```python
from build123d import *

# Parameters (mm, degrees)
F1_DEPTH  = 25
F2_R      = 4
F3_R      = 3.9581459444
F4_R      = 5
F6_DEPTH  = 4
F7_R      = 1
F9_DEPTH  = 10
F11_D     = 8.5
F11_DEPTH = 20
F11_TIP   = 2.5536576309
F13_D     = 10.3
F13_DEPTH = 4
F13_TIP   = 3.094432188
F15_D     = 10
F15_DEPTH = 4
F15_TIP   = 3.0043030951


with BuildPart() as f1:
    # F0 (on Front) → F1 (new body)
    with BuildSketch(Plane.XZ):
        Polygon((-11.592581531, 8.7356367638), (0, 0), (61, 0), (47.3139187714, 38.6483011348), (67.3029387003, 42.7151132025), (66.5054669627, 46.634812021), (42.0073493471, 41.6506136606), (55.3401309115, 4), (1.338381278, 4), (-10.3797117652, 12.8302164722), (-61.3117864463, 9.2686988641), (-61.0327605513, 5.278442663), align=None)
    extrude(amount=F1_DEPTH)

    # F2
    f2_edges = [f1.edges().sort_by_distance(p)[0] for p in [
        (42.007349, -12.5, 41.650614),
        (1.338381, -12.5, 4),
        (-10.379712, -12.5, 12.830216),
        (-11.592582, -12.5, 8.735637),
        (0, -12.5, 0),
        (47.313919, -12.5, 38.648301),
    ]]
    fillet(f2_edges, radius=F2_R)

    # F3
    f3_edges = [f1.edges().sort_by_distance(p)[0] for p in [
        (55.340131, -12.5, 4),
        (61, -12.5, 0),
    ]]
    fillet(f3_edges, radius=F3_R)

    # F4
    f4_edges = [f1.edges().sort_by_distance(p)[0] for p in [
        (66.904203, -25, 44.674963),
        (66.904203, 0, 44.674963),
    ]]
    fillet(f4_edges, radius=F4_R)

    # F5 (on face) → F6 (cut)
    with BuildSketch(Plane(origin=(-0.9433178269, 0, 13.4900734165), x_dir=(0.9975640503, 0, 0.0697564737), z_dir=(-0.0697564737, 0, 0.9975640503))):
        Polygon((-60.5158822671, 0), (-60.5158822671, -7.5), (-50.5158822671, -7.5), (-40.5158822671, 0), align=None)
        Polygon((-50.5158822671, -17.5), (-60.5158822671, -17.5), (-60.5158822671, -25), (-40.5158822671, -25), align=None)
    extrude(amount=-F6_DEPTH, mode=Mode.SUBTRACT)

    # F7
    f7_edges = [f1.edges().sort_by_distance(p)[0] for p in [
        (-41.220992, -25, 8.6687),
        (-51.196633, -17.5, 7.971136),
        (-61.172273, -17.5, 7.273571),
        (-61.172273, -7.5, 7.273571),
        (-41.220992, 0, 8.6687),
        (-51.196633, -7.5, 7.971136),
    ]]
    fillet(f7_edges, radius=F7_R)

    # F8 (on face) → F9 (join)
    with BuildSketch(Plane(origin=(-0.9433178269, 0, 13.4900734165), x_dir=(0.9975640503, 0, 0.0697564737), z_dir=(-0.0697564737, 0, 0.9975640503))):
        Polygon((-36.7410970494, -19.5), (-32.6996451651, -12.5), (-36.7410970494, -5.5), (-44.8240008181, -5.5), (-48.8654527024, -12.5), (-44.8240008181, -19.5), align=None)
    extrude(amount=F9_DEPTH)

    # F11
    with Locations(Plane(origin=(-1.6408825643, 0, 23.4657139191), x_dir=(0.9975640503, 0, 0.0697564737), z_dir=(-0.0697564737, 0, 0.9975640503))):
        with Locations((-40.7825489337, -12.5)):
            Hole(F11_D / 2, depth=F11_DEPTH)
            with Locations((0, 0, -(F11_DEPTH + F11_TIP / 2))):  # 118° drill point
                Cone(0, F11_D / 2, F11_TIP, mode=Mode.SUBTRACT)

    # F13
    with Locations(Plane(origin=(-0.6642919319, 0, 9.4998172155), x_dir=(0.9975640503, 0, 0.0697564737), z_dir=(0.0697564737, 0, -0.9975640503))):
        with Locations((-40.7825489337, 12.5)):
            Hole(F13_D / 2, depth=F13_DEPTH)
            with Locations((0, 0, -(F13_DEPTH + F13_TIP / 2))):  # 118° drill point
                Cone(0, F13_D / 2, F13_TIP, mode=Mode.SUBTRACT)

    # F15
    with Locations(Plane(origin=(-6.4674054427, 0, 31.7883133346), x_dir=(0.9799247046, 0, 0.1993679344), z_dir=(-0.1993679344, 0, 0.9799247046))):
        with Locations((64.4678362136, -14)):
            Hole(F15_D / 2, depth=F15_DEPTH)
            with Locations((0, 0, -(F15_DEPTH + F15_TIP / 2))):  # 118° drill point
                Cone(0, F15_D / 2, F15_TIP, mode=Mode.SUBTRACT)


solid = f1.part
```
CAD build for the part. Positions are in the model's coordinates, mm. A direction names the side the tool comes from. Coordinates: 2 decimals unless noted, no trailing zeros. Order: outer loops, then holes, each group sorted by start corner. A loop starts at its lowest first (then second) coordinate and runs counter-clockwise, first axis right, second up. Notation, with made-up numbers: (-17, -24) -> (25, -24) arc R22 cw to (25, 1) -> close; hole circle Ø7 at (-13, -38). An arc over 180 degrees is marked (long way). Use one line per item in the form item = value. Start each with the question number.
1) Drop flat-ended pins along their axis: pin 1 (1.4 mm diameter, centred on x = -54, z = 8, fed in from -Y); pin 2 (3 mm diameter, centred on y = -18.5, z = 30.5, fed in from +X); pin 3 (12 mm diameter, centred on y = -12.5, z = 41.5, fed in from -X). Give the stop position or say it passes through.
2) Pull direction X, two halves, no side cores. Call faces 6 (the flat face through (-56, -7.5, 8)), 7 (the cylindrical face through (43.856, -12.675, 40.66)), 8 (the cylindrical face through (-45.906, -14.128, 15.563)): +X half, -X half, draft (parallel to the pull), parting line (faces both ways), or undercut.
3) Band-saw the part on B-B on y = -22. Give the cut face in (x, z), then the cut area to 3 significant figures.
4) Tool access for faces 1 (the cylindrical face through (1.425, -12.675, 4.201)), 2 (the flat face through (-48.046, -15.951, 15.138)), 3 (the flat face through (-42, -5.5, 16)), 4 (the flat face through (-5.8, -12.32, 4.37)), 5 (the flat face through (54.062, -12.325, 19.592)): list every direction of +Z, -Z, +X, -X, +Y, -Y with a clear straight run to the whole face (end or side of a thin tool).
5) Band-saw the part on C-C on x = 31.5. Give the cut face in (y, z), then the cut area to 3 significant figures.
6) Drill centre lines: L1, parallel to X at y = -9.5, z = 17.5; L2, parallel to X at y = -7.5, z = 19.5; L3, parallel to Z at x = 39.5, y = -23.25. Where is each one in solid material? Low to high. Write a range as [from, to].
7) Band-saw the part on D-D on y = -3.5. Give the cut face in (x, z).
8) Band-saw the part on A-A on z = 15. State how many separate pieces and enclosed holes the cut face has, then the cut area to 3 significant figures.
Entries:
q1.pin_1 = -17.5
q1.pin_2 = 50.73
q1.pin_3 = 43.31
q2.face_6 = draft
q2.face_7 = -X half
q2.face_8 = undercut
q3.outline = (-45.35, 10.38) -> (-45.07, 6.39) -> (-13.08, 8.63) arc R4 cw to (-10.4, 7.84) -> (-1.07, 0.81) arc R4 ccw to (1.34, 0) -> (55.4, 0) arc R3.96 ccw to (59.13, 5.28) -> (48.85, 34.31) arc R4 cw to (51.82, 39.57) -> (66.89, 42.63) -> (66.1, 46.55) -> (46.52, 42.57) arc R4 ccw to (43.54, 37.31) -> (53.47, 9.28) arc R3.96 cw to (49.74, 4) -> (2.68, 4) arc R4 cw to (0.27, 4.81) -> (-9.19, 11.93) arc R4 ccw to (-11.87, 12.73) -> close
q3.area = 677 mm2
q4.face_1 = +Z, +Y, -Y
q4.face_2 = -X, -Y
q4.face_3 = +Z, -X, +Y
q4.face_4 = -Z, +Y, -Y
q4.face_5 = +X, +Y, -Y
q5.outline = (-25, 0) -> (0, 0) -> (0, 4) -> (-25, 4) -> close
q5.area = 100 mm2
q6.L1 = [-48.47, -45.12], [-39.09, -35.74], [50.56, 54.8]
q6.L2 = [-47.45, -37.04], [49.85, 54.09]
q6.L3 = [0, 4]
q7.outline = (-46.02, 10.34) -> (-45.74, 6.35) -> (-13.08, 8.63) arc R4 cw to (-10.4, 7.84) -> (-1.07, 0.81) arc R4 ccw to (1.34, 0) -> (55.4, 0) arc R3.96 ccw to (59.13, 5.28) -> (48.85, 34.31) arc R4 cw to (51.82, 39.57) -> (67.08, 42.67) -> (66.28, 46.59) -> (46.52, 42.57) arc R4 ccw to (43.54, 37.31) -> (53.47, 9.28) arc R3.96 cw to (49.74, 4) -> (2.68, 4) arc R4 cw to (0.27, 4.81) -> (-9.19, 11.93) arc R4 ccw to (-11.87, 12.73) -> close
q8.separate_pieces = 2
q8.enclosed_holes = 1
q8.area = 219 mm2
